from build123d import *

# Parameters (mm, degrees)
F0_W     = 4.5
F0_H     = 1
F1_DEPTH = 5.8
F2_R     = 4.25
F3_DEPTH = 4.1
F5_D     = 3


with BuildPart() as f1:
    # F0 (on Top) → F1 (new body, symmetric)
    with BuildSketch(Plane.XY):
        Polygon((11.4, 0), (-11.4, 0), (-11.4, -4), (-11.4, -5), (-11.4, -19.5), (11.4, -19.5), (11.4, -5), (11.4, -4), align=None)
        with Locations((-13.65, -4.5)):
            Rectangle(F0_W, F0_H)
        with Locations((13.65, -4.5)):
            Rectangle(F0_W, F0_H)
    extrude(amount=F1_DEPTH, both=True)

    # F2 (on face) → F3 (join)
    with BuildSketch(Plane(origin=(0, 0, 0), x_dir=(-1, 0, 0), z_dir=(0, 1, 0))):
        with Locations((7.1, 0)):
            Circle(F2_R)
    extrude(amount=F3_DEPTH)

    # F5 (through all)
    with Locations(Plane(origin=(0, 0, 0), x_dir=(1, 0, 0), z_dir=(0, 1, 0))):
        with Locations((14.15, 0), (-14.15, 0)):
            Hole(F5_D / 2)


solid = f1.part
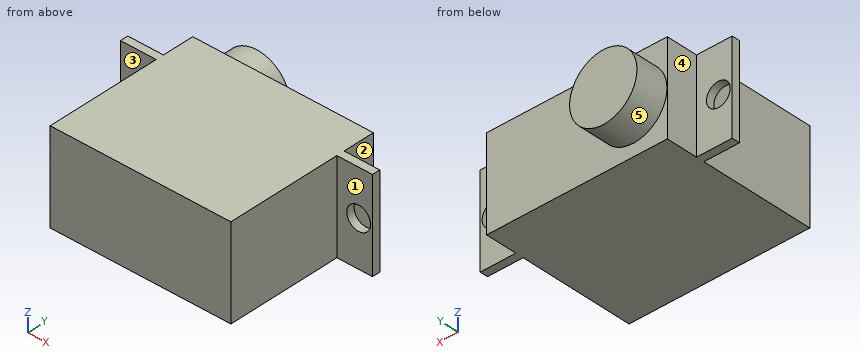
Here's how the part is built. I have some questions about the finished solid (model axes, mm). Face numbers are marked on the shaded views. A direction names the side the tool comes from. Coordinates: 2 decimals unless noted, no trailing zeros. Order: outer loops, then holes, each group sorted by start corner. A loop starts at its lowest first (then second) coordinate and runs counter-clockwise, first axis right, second up. Notation, with made-up numbers: (-15.5, 36.25) -> (41.5, 36.25) arc R16 ccw to (41.5, 67.25) -> close; hole circle Ø5 at (27.25, 15). An arc over 180 degrees is marked (long way). Answer in a Markdown table with one row per item.
(1) I want a section at D-D on y = -5.5. List the corners of the cut face in (x, z) for me.
Answer key:
| item | result |
|---|---|
| outline | (-11.4, -5.8) -> (11.4, -5.8) -> (11.4, 5.8) -> (-11.4, 5.8) -> close |
(2) I want a section at A-A on x = 14.15. List the corners of the cut face in (y, z) for me.
Answer key:
| item | result |
|---|---|
| outline | (-5, -5.8) -> (-4, -5.8) -> (-4, -1.5) -> (-5, -1.5) -> close; (-5, 1.5) -> (-4, 1.5) -> (-4, 5.8) -> (-5, 5.8) -> close |
(3) I want a section at C-C on z = -3.75. List the corners of the cut face in (x, y) for me.
Answer key:
| item | result |
|---|---|
| outline | (-15.9, -5) -> (-11.4, -5) -> (-11.4, -19.5) -> (11.4, -19.5) -> (11.4, -5) -> (15.9, -5) -> (15.9, -4) -> (11.4, -4) -> (11.4, 0) -> (-5.1, 0) -> (-5.1, 4.1) -> (-9.1, 4.1) -> (-9.1, 0) -> (-11.4, 0) -> (-11.4, -4) -> (-15.9, -4) -> close |
(4) I want a section at B-B on z = 0. List the corners of the cut face in (x, y) for me.
Answer key:
| item | result |
|---|---|
| outline | (-15.9, -5) -> (-15.65, -5) -> (-15.65, -4) -> (-15.9, -4) -> close; (-12.65, -5) -> (-11.4, -5) -> (-11.4, -19.5) -> (11.4, -19.5) -> (11.4, -5) -> (12.65, -5) -> (12.65, -4) -> (11.4, -4) -> (11.4, 0) -> (-2.85, 0) -> (-2.85, 4.1) -> (-11.35, 4.1) -> (-11.35, 0) -> (-11.4, 0) -> (-11.4, -4) -> (-12.65, -4) -> close; (15.65, -5) -> (15.9, -5) -> (15.9, -4) -> (15.65, -4) -> close |
(5) Please list where these lines run through material, in increasing order: probe 1 along Z at (x, y) = (-14.15, -4.45); probe 2 along Y at (x, z) = (3, -4.25); probe 3 along X at (y, z) = (-4.5, -0.75).
Answer key:
| item | result |
|---|---|
| probe 1 | -5.8 to -1.5, 1.5 to 5.8 |
| probe 2 | -19.5 to 0 |
| probe 3 | -15.9 to -15.45, -12.85 to 12.85, 15.45 to 15.9 |
(6) Will these pins go through, and if not, where does the flat tip stop? pin 1 Ø3.5 at (x, z) = (-14.5, 2.5) entering from -Y; pin 2 Ø2 at (x, z) = (-13, -2.5) entering from +Y; pin 3 Ø6 at (y, z) = (-9, 2) entering from +X.
Answer key:
| item | result |
|---|---|
| pin 1 | y = -5 |
| pin 2 | y = -4 |
| pin 3 | x = 11.4 |
(7) On a 3-axis mill with a long thin cutter (end or side, diameter ignored), from which of +Z, -Z, +X, -X, +Y, -Y can I reach the whole of each face in a straight line? I mean the marked faces 1, 2, 3, 4 and 5. Say none if no direction works.
Answer key:
| item | result |
|---|---|
| face 1 | +Z, -Z, +X, -Y |
| face 2 | +Z, -Z, +X, +Y |
| face 3 | +Z, -Z, -X, -Y |
| face 4 | +Z, -Z, -X, +Y |
| face 5 | +Y |
